from build123d import *

# Parameters (mm, degrees)
F0_W      = 64
F0_H      = 28
F0_W_2    = 14
F0_H_2    = 9.8
F0_R      = 4
F1_DEPTH  = 5
F1_FACE_W = 64
F1_FACE_H = 10
F4_DEPTH  = 1.2
F5_DEPTH  = 1.2
F7_D      = 3.1
F7_DEPTH  = 15
F7_TIP    = 0.9313339595
F8_R      = 2.75
F9_DEPTH  = 5.5
F10_R     = 1.55
F11_DEPTH = 5
F12_DEPTH = 11.5
F13_R     = 3


# Not quite as in the source:
# - a pattern or mirror of a feature is missing from the dataset's text; its kind, count and spacing are read off the source's solid


with BuildPart() as f1:
    # F0 (on Front) → F1 (new body, symmetric)
    with BuildSketch(Plane.XZ):
        Rectangle(F0_W, F0_H)
        with Locations((0, -2.4)):
            Rectangle(F0_W_2, F0_H_2, mode=Mode.SUBTRACT)
        with Locations((-21.5, 6)):
            Circle(F0_R, mode=Mode.SUBTRACT)
        with Locations((21.5, 6)):
            Circle(F0_R, mode=Mode.SUBTRACT)
    extrude(amount=F1_DEPTH, both=True)

    # F3 (on offset) + F1_face (on face) → F4 (cut, symmetric)
    with BuildSketch(Plane(origin=(0, 0, -4), x_dir=(1, 0, 0), z_dir=(0, 0, -1))):
        Polygon((18.75, 1.5877132403), (18.75, -1.5877132403), (18.75, -5), (24.25, -5), (24.25, 1.5877132403), (21.5, 3.1754264805), align=None)
    with BuildSketch(Plane(origin=(0, 0, -14), x_dir=(1, 0, 0), z_dir=(0, 0, -1))):
        Rectangle(F1_FACE_W, F1_FACE_H)
    extrude(amount=F4_DEPTH, both=True, mode=Mode.SUBTRACT)

    # F3 (on offset) → F5 (cut, symmetric)
    with BuildSketch(Plane(origin=(0, 0, -4), x_dir=(1, 0, 0), z_dir=(0, 0, -1))):
        Polygon((18.75, 1.5877132403), (18.75, -1.5877132403), (18.75, -5), (24.25, -5), (24.25, 1.5877132403), (21.5, 3.1754264805), align=None)
    f5 = extrude(amount=F5_DEPTH, both=True, mode=Mode.SUBTRACT)

    # F5_copies: F5 across plane
    add(f5.mirror(Plane(origin=(0, 0, 0), x_dir=(0, 0, -1), z_dir=(-1, 0, 0))), mode=Mode.SUBTRACT)

    # F7
    with Locations(Plane(origin=(0, 0, -12.8), x_dir=(1, 0, 0), z_dir=(0, 0, -1))):
        with Locations((21.5, 0), (-21.5, 0)):
            Hole(F7_D / 2, depth=F7_DEPTH)
            with Locations((0, 0, -(F7_DEPTH + F7_TIP / 2))):  # 118° drill point
                Cone(0, F7_D / 2, F7_TIP, mode=Mode.SUBTRACT)

    # F8 (on face) → F9 (cut, through all)
    with BuildSketch(Plane(origin=(0, 0, -12.8), x_dir=(1, 0, 0), z_dir=(0, 0, -1))):
        Circle(F8_R)
    extrude(amount=-F9_DEPTH, mode=Mode.SUBTRACT)

    # F10 (on face) → F11 (cut)
    with BuildSketch(Plane.XY.offset(14)):
        Polygon((-1.5877132403, -2.75), (1.5877132403, -2.75), (3.1754264805, 0), (1.5877132403, 2.75), (-1.5877132403, 2.75), (-3.1754264805, 0), align=None)
        Circle(F10_R, mode=Mode.SUBTRACT)
    extrude(amount=-F11_DEPTH, mode=Mode.SUBTRACT)

    # F12 (cut, through all): a face of the model
    f12_faces = [f1.faces().sort_by_distance(p)[0] for p in [
        (0, 0, 14),
    ]]
    extrude(f12_faces, amount=-F12_DEPTH, mode=Mode.SUBTRACT)

    # F13
    f13_edges = [f1.edges().sort_by_distance(p)[0] for p in [
        (32, 0, 14),
        (-32, 0, 14),
        (32, 0, -12.8),
        (-32, 0, -12.8),
    ]]
    fillet(f13_edges, radius=F13_R)


solid = f1.part
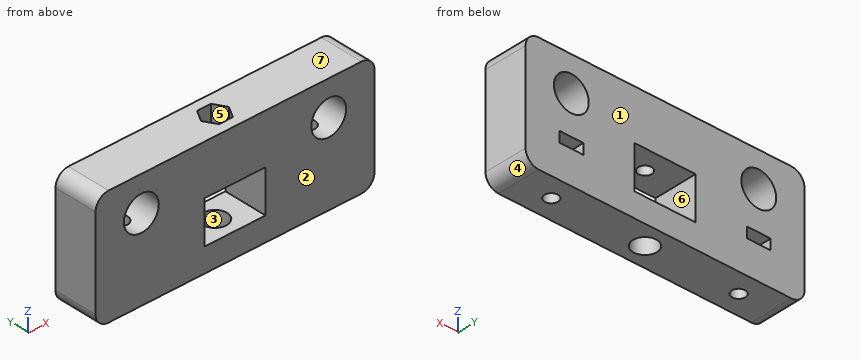
Read the model definition and answer for the solid it produces. Units are mm, in the model's axes. Face numbers are marked on the shaded views. A direction names the side the tool comes from. Round coordinates to 2 decimals unless told otherwise and drop trailing zeros. Order: outer loops, then holes, each group sorted by start corner. A loop starts at its lowest first (then second) coordinate and runs counter-clockwise, first axis right, second up. Notation, with made-up numbers: (78.25, -18) - (109.25, -18) arc R36 cw to (109.25, 21) - close; hole circle Ø9 at (20, 6.5). An arc over 180 degrees is marked (long way). Use one line per item in the form item = value. Start each with the question number.
(1) Flat-ended cylindrical pins translate along their axes: pin 1 Ø2.5 at (x, y) = (21.5, 0) entering from -Z; pin 2 Ø5 at (x, y) = (0, 0) entering from -Z. Find the tip coordinate at first contact, or state that the pin passes through.
(2) The part is cut by section C-C (z = 11.75). Give the vertices of the cut face in (x, y).
(3) For the marked faces 5, 6 and 7, determine the directions among +Z, -Z, +X, -X, +Y, -Y from which every point of the face is accessible in a straight line to the end or side of a thin tool.
(4) Determine the mould class of the marked faces 1, 2, 3 and 4 for opening direction Y: +Y half, -Y half, draft (parallel to the pull), parting line (faces both ways), or undercut.
(5) The part is cut by section A-A (z = 6). Give the vertices of the cut face in (x, y), then the cut area to 3 significant figures.
(6) The part is cut by section B-B (x = -4.5). Give the vertices of the cut face in (y, z).
(7) Find the intervals of material crossed by line 1 along X through (y, z) = (-2, 0); line 2 along Y through (x, z) = (21.5, 0.5); line 3 along X through (y, z) = (-2.5, 3), in increasing order. Write a range as from..to.
Checked values:
q1.pin_1 = 9.8
q1.pin_2 = 2.5
q2.outline = (-31.9, -5) - (31.9, -5) - (31.9, 5) - (-31.9, 5) - close; hole (-3.18, 0) - (-1.59, -2.75) - (1.59, -2.75) - (3.18, 0) - (1.59, 2.75) - (-1.59, 2.75) - close
q3.face_5 = +Z
q3.face_6 = +Y, -Y
q3.face_7 = +Z, +X, -X, +Y, -Y
q4.face_1 = +Y half
q4.face_2 = -Y half
q4.face_3 = undercut
q4.face_4 = draft
q5.outline = (-32, -5) - (-25.5, -5) - (-25.5, 5) - (-32, 5) - close; (-17.5, -5) - (17.5, -5) - (17.5, 5) - (-17.5, 5) - close; (25.5, -5) - (32, -5) - (32, 5) - (25.5, 5) - close; hole circle Ø3.1 at (0, 0)
q5.area = 472 mm^2
q6.outline = (-5, -12.8) - (5, -12.8) - (5, -7.3) - (-5, -7.3) - close; (-5, 2.5) - (5, 2.5) - (5, 14) - (-5, 14) - close
q7.line_1 = -32..-7, 7..32
q7.line_2 = -5..-1.55, 1.55..5
q7.line_3 = -32..-24.15, -18.85..18.85, 24.15..32
